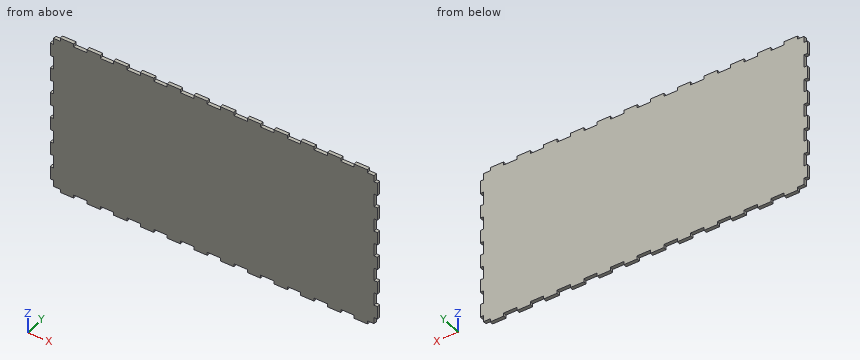
from build123d import *

# Parameters (mm, degrees)
BOSS_EXTRUDE1_DEPTH = 6.35


with BuildPart() as part:
    # Sketch2 → Boss-Extrude1 (new body)
    with BuildSketch(Plane(origin=(0, 0, 0), x_dir=(1, 0, 0), z_dir=(0, 1, 0))):
        Polygon((-292.1, 152.4), (-292.1, 158.75), (-266.7, 158.75), (-266.7, 152.4), (-241.3, 152.4), (-241.3, 158.75), (-215.9, 158.75), (-215.9, 152.4), (-190.5, 152.4), (-190.5, 158.75), (-165.1, 158.75), (-165.1, 152.4), (-139.7, 152.4), (-139.7, 158.75), (-114.3, 158.75), (-114.3, 152.4), (-88.9, 152.4), (-88.9, 158.75), (-63.5, 158.75), (-63.5, 152.4), (-38.1, 152.4), (-38.1, 158.75), (-12.7, 158.75), (-12.7, 152.4), (12.7, 152.4), (12.7, 158.75), (38.1, 158.75), (38.1, 152.4), (63.5, 152.4), (63.5, 158.75), (88.9, 158.75), (88.9, 152.4), (114.3, 152.4), (114.3, 158.75), (139.7, 158.75), (139.7, 152.4), (165.1, 152.4), (165.1, 158.75), (190.5, 158.75), (190.5, 152.4), (215.9, 152.4), (215.9, 158.75), (241.3, 158.75), (241.3, 152.4), (266.7, 152.4), (266.7, 158.75), (292.1, 158.75), (292.1, 152.4), (304.8, 152.4), (304.8, 139.7), (311.15, 139.7), (311.15, 114.3), (304.8, 114.3), (304.8, 88.9), (311.15, 88.9), (311.15, 63.5), (304.8, 63.5), (304.8, 38.1), (311.15, 38.1), (311.15, 12.7), (304.8, 12.7), (304.8, -12.7), (311.15, -12.7), (311.15, -38.1), (304.8, -38.1), (304.8, -63.5), (311.15, -63.5), (311.15, -88.9), (304.8, -88.9), (304.8, -114.3), (311.15, -114.3), (311.15, -139.7), (304.8, -139.7), (304.8, -152.4), (292.1, -152.4), (292.1, -158.75), (266.7, -158.75), (266.7, -152.4), (241.3, -152.4), (241.3, -158.75), (215.9, -158.75), (215.9, -152.4), (190.5, -152.4), (190.5, -158.75), (165.1, -158.75), (165.1, -152.4), (139.7, -152.4), (139.7, -158.75), (114.3, -158.75), (114.3, -152.4), (88.9, -152.4), (88.9, -158.75), (63.5, -158.75), (63.5, -152.4), (38.1, -152.4), (38.1, -158.75), (12.7, -158.75), (12.7, -152.4), (-12.7, -152.4), (-12.7, -158.75), (-38.1, -158.75), (-38.1, -152.4), (-63.5, -152.4), (-63.5, -158.75), (-88.9, -158.75), (-88.9, -152.4), (-114.3, -152.4), (-114.3, -158.75), (-139.7, -158.75), (-139.7, -152.4), (-165.1, -152.4), (-165.1, -158.75), (-190.5, -158.75), (-190.5, -152.4), (-215.9, -152.4), (-215.9, -158.75), (-241.3, -158.75), (-241.3, -152.4), (-266.7, -152.4), (-266.7, -158.75), (-292.1, -158.75), (-292.1, -152.4), (-304.8, -152.4), (-304.8, -139.7), (-311.15, -139.7), (-311.15, -114.3), (-304.8, -114.3), (-304.8, -88.9), (-311.15, -88.9), (-311.15, -63.5), (-304.8, -63.5), (-304.8, -38.1), (-311.15, -38.1), (-311.15, -12.7), (-304.8, -12.7), (-304.8, 12.7), (-311.15, 12.7), (-311.15, 38.1), (-304.8, 38.1), (-304.8, 63.5), (-311.15, 63.5), (-311.15, 88.9), (-304.8, 88.9), (-304.8, 114.3), (-311.15, 114.3), (-311.15, 139.7), (-304.8, 139.7), (-304.8, 152.4), align=None)
    extrude(amount=BOSS_EXTRUDE1_DEPTH)


solid = part.part
CAD build for the part. Positions are in the model's coordinates, mm. Coordinates: 2 decimals unless noted, no trailing zeros. Loops run counter-clockwise (first coordinate to the right, second up) from the corner with the lowest first, then second, coordinate; pieces in that order, holes last. Notation, with made-up numbers: (10, -2.75) - (26, -2.75) arc R32 cw to (26, 27.25) - close; hole circle Ø7 at (-22.5, -22.5). An arc over 180 degrees is marked (long way). Use one line per item in the form item = value. Start each with the question number.
1) Band-saw the part on A-A (z = -4.5). Give the cut face in (x, y), and give its area (3 significant figures).
2) Flat gauge pins, fed straight in: pin 1 (1.9 mm diameter, centred on y = 3, z = 157, fed in from -X); pin 2 (3 mm diameter, centred on y = 1.5, z = -157, fed in from +X); pin 3 (1.9 mm diameter, centred on x = -55, y = 2, fed in from +Z). Where does each tip first touch, or does it go through?
3) Drill centre lines: L1, parallel to Z at x = -54.5, y = 4; L2, parallel to X at y = 3.75, z = 43. Where is each one in solid material? Low to high. Write a range as from..to.
4) Band-saw the part on B-B (x = 260). Give the cut face in (y, z).
Check values:
q1.outline = (-304.8, 0) - (304.8, 0) - (304.8, 6.35) - (-304.8, 6.35) - close
q1.area = 3,870 mm2
q2.pin_1 = -292.1
q2.pin_2 = 292.1
q2.pin_3 = 152.4
q3.L1 = -152.4..152.4
q3.L2 = -304.8..304.8
q4.outline = (0, -152.4) - (6.35, -152.4) - (6.35, 152.4) - (0, 152.4) - close
